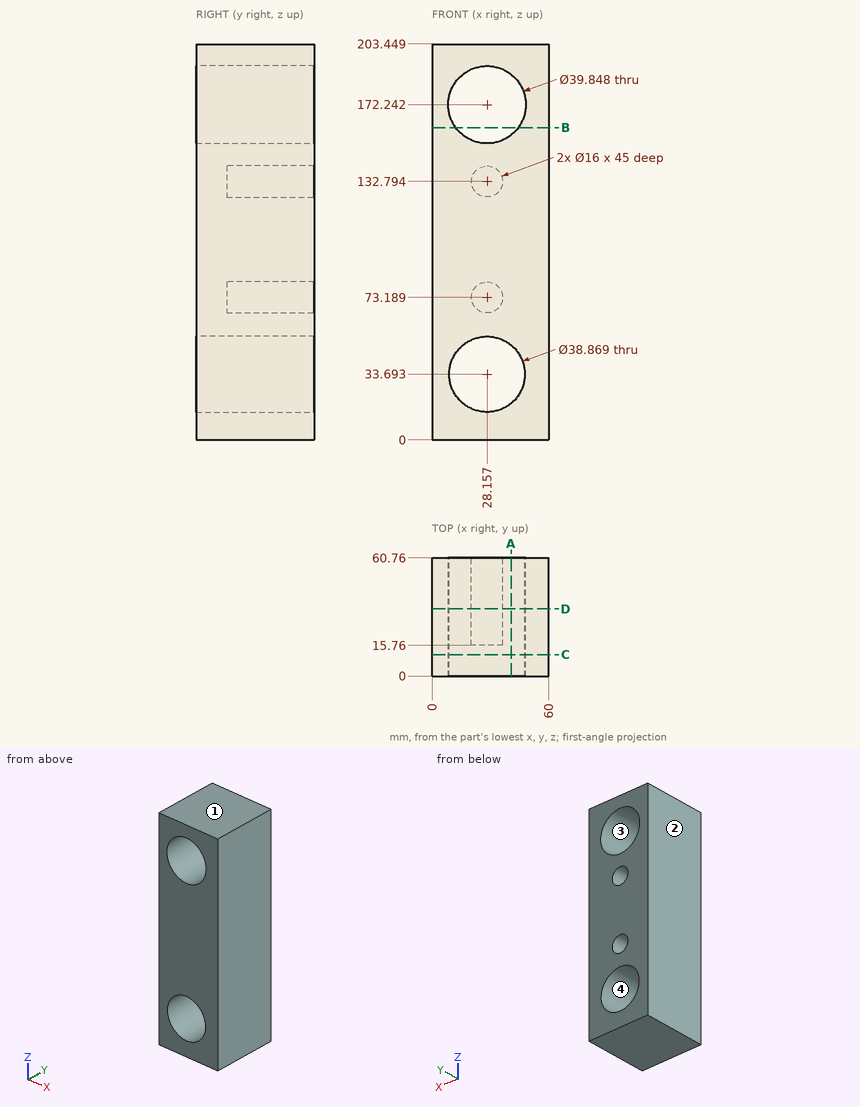
Drawing for the job (mm, zero at the part's lowest x, y, z). Give positions to 0.01 mm unless a question says otherwise; leave off trailing zeros. Order: outer loops, then holes, each group sorted by start corner. A loop starts at its lowest first (then second) coordinate and runs counter-clockwise, first axis right, second up. Notation, with made-up numbers: M -32,27.25 L 27,27.25 A27 ccw 27,44.25 Z; hole C 22.5,-23.5 d5. An arc over 180 degrees is marked long. Use a Markdown table: item, result. Add a question column.
(1) Probe line 1 along X through (y, z) = (39, 34) (1 decimal); line 2 along Z through (x, y) = (27, 42) (1 decimal); line 3 along X through (y, z) = (47.5, 173). List the from-to ranges inside material, lowest first. Write a range as [from, to].
(2) Mould opens along X. For the marked faces 1, 2, 3 and 4 say: +X half, -X half, draft (parallel to the pull), parting line (faces both ways), or undercut.
(3) Saw through at C-C, the plane y = 11. Give the cut face in (x, z) (1 decimal).
(4) Saw through at A-A, the plane x = 40.5. Give the cut face in (y, z) (1 decimal).
(5) Drop a flat-ended pin along its axis: P1, Ø5, axis at x = 25.5, z = 136, coming from the +Y side. Give the stop position or say it passes through.
(6) Saw through at D-D, the plane y = 34.5. Give the cut face in (x, z) (1 decimal).
(7) Saw through at B-B, the plane z = 160.5. Give the cut face in (x, y), and give its area (3 significant figures).
Answer key:
| question | item | result |
|---|---|---|
| 1 | line 1 | [0, 8.7], [47.6, 60] |
| 1 | line 2 | [0, 14.3], [53.1, 65.3], [81.1, 124.9], [140.7, 152.4], [192.1, 203.4] |
| 1 | line 3 | [0, 8.25], [48.07, 60] |
| 2 | face 1 | draft |
| 2 | face 2 | -X half |
| 2 | face 3 | undercut |
| 2 | face 4 | undercut |
| 3 | outline | M 0,0 L 60,0 L 60,203.4 L 0,203.4 Z; hole C 28.2,172.2 d39.8; hole C 28.2,33.7 d38.9 |
| 4 | outline | M 0,0 L 60.8,0 L 60.8,18.7 L 0,18.7 Z; M 0,48.7 L 60.8,48.7 L 60.8,156.6 L 0,156.6 Z; M 0,187.9 L 60.8,187.9 L 60.8,203.4 L 0,203.4 Z |
| 5 | P1 | y = 15.76 |
| 6 | outline | M 0,0 L 60,0 L 60,203.4 L 0,203.4 Z; hole C 28.2,172.2 d39.8; hole C 28.2,33.7 d38.9; hole C 28.2,73.2 d16; hole C 28.2,132.8 d16 |
| 7 | outline | M 0,0 L 12.06,0 L 12.06,60.76 L 0,60.76 Z; M 44.25,0 L 60,0 L 60,60.76 L 44.25,60.76 Z |
| 7 | area | 1,690 mm^2 |
